```python
from build123d import *

# Parameters (mm, degrees)
SKETCH1_W           = 31.75
SKETCH1_H           = 72.39
BOSS_EXTRUDE1_DEPTH = 3.175
SKETCH3_W           = 15.24
SKETCH3_H           = 35.814
CUT_EXTRUDE1_DEPTH  = 3.175
SKETCH4_W           = 3.81
SKETCH4_H           = 3.81
SKETCH4_R           = 1.905
CUT_EXTRUDE9_DEPTH  = 3.175


with BuildPart() as part:
    # Sketch1 → Boss-Extrude1 (new body)
    with BuildSketch(Plane(origin=(0, 0, 0), x_dir=(1, 0, 0), z_dir=(0, 1, 0))):
        Rectangle(SKETCH1_W, SKETCH1_H)
    extrude(amount=BOSS_EXTRUDE1_DEPTH)

    # Sketch3 → Cut-Extrude1 (cut)
    with BuildSketch(Plane(origin=(0, 3.175, 0), x_dir=(1, 0, 0), z_dir=(0, 1, 0))):
        Rectangle(SKETCH3_W, SKETCH3_H)
    extrude(amount=-CUT_EXTRUDE1_DEPTH, mode=Mode.SUBTRACT)

    # Sketch4 → Cut-Extrude9 (cut)
    with BuildSketch(Plane(origin=(0, 3.175, 0), x_dir=(1, 0, 0), z_dir=(0, 1, 0))):
        Polygon((-3.81, 23.622), (-3.81, 17.907), (3.81, 17.907), (3.81, 23.622), (1.905, 23.622), (-1.905, 23.622), align=None)
        with Locations((0, 25.527)):
            Rectangle(SKETCH4_W, SKETCH4_H)
        with Locations(Location((-3.81, -21.209, 0), (0, 0, 270))):
            Circle(SKETCH4_R)
    extrude(amount=-CUT_EXTRUDE9_DEPTH, mode=Mode.SUBTRACT)


solid = part.part
```
Build history of the part. All positions in model axes, mm. A direction names the side the tool comes from. Coordinates: 2 decimals unless noted, no trailing zeros. Order: outer loops, then holes, each group sorted by start corner. A loop starts at its lowest first (then second) coordinate and runs counter-clockwise, first axis right, second up. Notation, with made-up numbers: (-25.5, 82.5) -> (-5.5, 82.5) arc R22 cw to (-5.5, 96.5) -> close; hole circle Ø6 at (56, 31.5). An arc over 180 degrees is marked (long way). Answer in a Markdown table with one row per item. Add a question column.
Q1. Band-saw the part on A-A, the plane z = -26. List the corners of the cut face in (x, y) (3 decimals), then the cut area to 3 significant figures.
Q2. Band-saw the part on C-C, the plane z = -1. List the corners of the cut face in (x, y) (3 decimals).
Q3. Mould opens along X. For faces 1 (the face through (-3.238, 1.61, 23.026)), 2 (the face through (-15.875, 2, 1)), 3 (the face through (15.875, 2, 1)) say: +X half, -X half, draft (parallel to the pull), parting line (faces both ways), or undercut.
Q4. Band-saw the part on B-B, the plane y = 2.2. List the corners of the cut face in (x, z) (3 decimals).
Q5. Which spindle directions (+Z, -Z, +X, -X, +Y, -Y) get a long thin tool onto all of the face, cutting with end or side? Do faces 4 (the face through (6, 2, -17.907)), 5 (the face through (0, 2, 36.195)). Say none if no direction does.
Q6. Wall check: line 1 along Z through (x, y) = (4.5, 1.3) (3 decimals); line 2 along X through (y, z) = (2.4, 15) (3 decimals); line 3 along Z through (x, y) = (1.5, 1.25) (3 decimals). Give the ranges that are in metal, low to high. Write a range as [from, to].
Answers follow:
| question | item | result |
|---|---|---|
| 1 | outline | (-15.875, 0) -> (-1.905, 0) -> (-1.905, 3.175) -> (-15.875, 3.175) -> close; (1.905, 0) -> (15.875, 0) -> (15.875, 3.175) -> (1.905, 3.175) -> close |
| 1 | area | 88.7 mm^2 |
| 2 | outline | (-15.875, 0) -> (-7.62, 0) -> (-7.62, 3.175) -> (-15.875, 3.175) -> close; (7.62, 0) -> (15.875, 0) -> (15.875, 3.175) -> (7.62, 3.175) -> close |
| 3 | face 1 | undercut |
| 3 | face 2 | -X half |
| 3 | face 3 | +X half |
| 4 | outline | (-15.875, -36.195) -> (15.875, -36.195) -> (15.875, 36.195) -> (-15.875, 36.195) -> close; hole (-7.62, -17.907) -> (-3.81, -17.907) -> (-3.81, -23.622) -> (-1.905, -23.622) -> (-1.905, -27.432) -> (1.905, -27.432) -> (1.905, -23.622) -> (3.81, -23.622) -> (3.81, -17.907) -> (7.62, -17.907) -> (7.62, 17.907) -> (-7.62, 17.907) -> close; hole circle Ø3.81 at (-3.81, 21.209) |
| 5 | face 4 | +Y, -Y |
| 5 | face 5 | +Z, +X, -X, +Y, -Y |
| 6 | line 1 | [-36.195, -17.907], [17.907, 36.195] |
| 6 | line 2 | [-15.875, -7.62], [7.62, 15.875] |
| 6 | line 3 | [-36.195, -27.432], [17.907, 36.195] |
